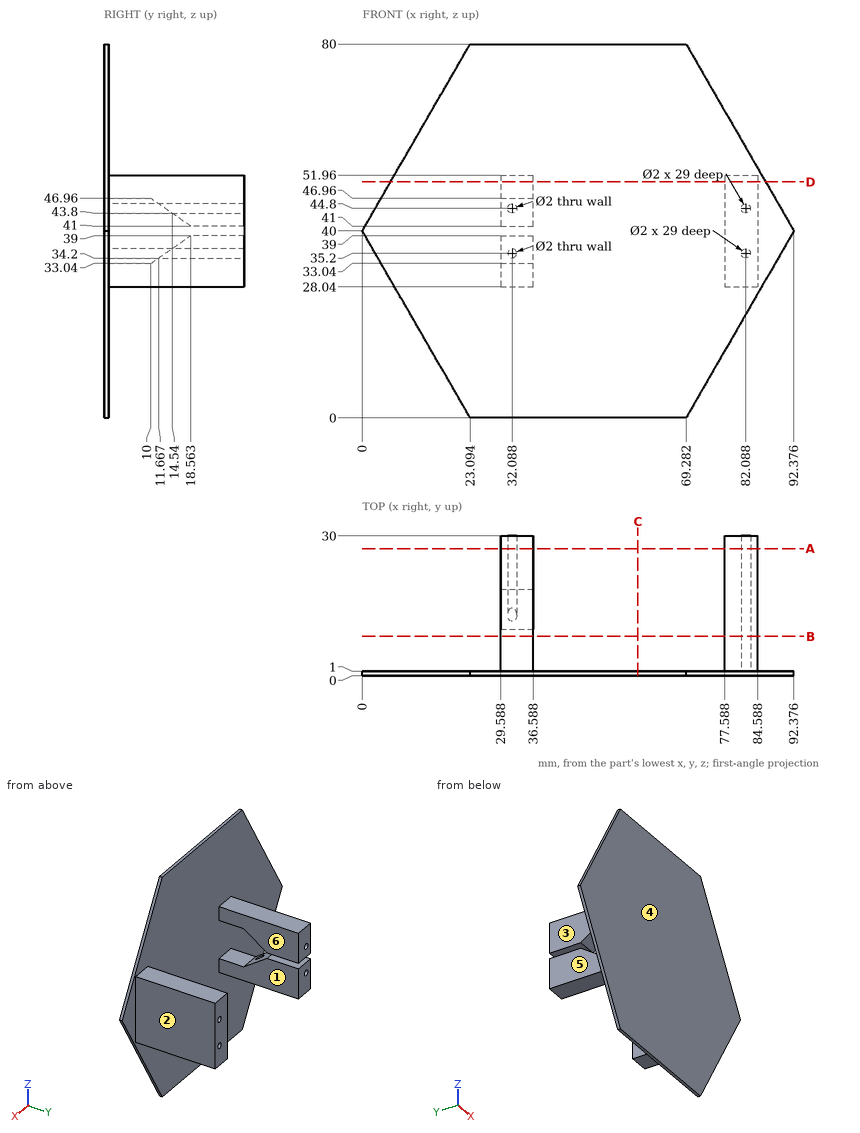
Input: dimensioned drawing with shaded views. Units: mm. Origin: part minimum x, y, z. A direction names the side the tool comes from. Give positions to 0.01 mm unless a question says otherwise; leave off trailing zeros. Write each loop counter-clockwise with the first axis right and the second up, starting at its lowest first coordinate (ties: lowest second). Pieces come first, ordered by that corner, then holes. Notation, with made-up numbers: (62, 24) -> (101, 24) arc R22 cw to (101, 43) -> close; hole circle Ø9 at (20.25, 43). An arc over 180 degrees is marked (long way). Return JSON: item names as keys, results as strings. Group by question number.
1. Pin query (flat end, axial travel): pin 1 Ø2.5 at (x, z) = (32.09, 44.8) entering from +Y; pin 2 Ø12 at (y, z) = (14.5, 37.5) entering from -X; pin 3 Ø3.5 at (x, y) = (34, 25) entering from +Z; pin 4 Ø12 at (y, z) = (10, 46.5) entering from +X. Return the tip coordinate at first contact, or that it passes through.
2. Section A-A, the plane y = 27.25. Output: boundary loops of the cut face in (x, z).
3. Section D-D, the plane z = 50.5. Output: boundary loops of the cut face in (x, y).
4. Access query for the marked faces 4, 5 and 6. Directions: +Z, -Z, +X, -X, +Y, -Y. A direction counts if a zero-diameter tool reaches every point of the face in a straight line with its end or side. Return the directions, or none.
5. Material intervals for line 1 (X direction, y = 13.5, z = 44.8); line 2 (Z direction, x = 36.5, y = 25.5); line 3 (X direction, y = 8.25, z = 35.2), sorted ascending. Write a range as from..to.
6. Section B-B, the plane y = 8.5. Output: boundary loops of the cut face in (x, z).
7. Mould query, pull axis X, two halves, no side actions, for the marked faces 1, 2 and 3. Classes: +X half, -X half, draft (parallel to the pull), parting line (faces both ways), or undercut.
8. Section C-C, the plane x = 59. Output: boundary loops of the cut face in (y, z).
Determined:
{
 "1": {"pin 1": "stops at y = 30", "pin 2": "stops at x = 29.59", "pin 3": "stops at z = 51.96", "pin 4": "stops at x = 84.59"},
 "2": {"outline": "(29.59, 28.04) -> (36.59, 28.04) -> (36.59, 39) -> (29.59, 39) -> close; (29.59, 41) -> (36.59, 41) -> (36.59, 51.96) -> (29.59, 51.96) -> close; (77.59, 28.04) -> (84.59, 28.04) -> (84.59, 51.96) -> (77.59, 51.96) -> close; hole circle Ø2 at (32.09, 35.2); hole circle Ø2 at (32.09, 44.8); hole circle Ø2 at (82.09, 35.2); hole circle Ø2 at (82.09, 44.8)"},
 "3": {"outline": "(6.06, 0) -> (86.31, 0) -> (86.31, 1) -> (84.59, 1) -> (84.59, 30) -> (77.59, 30) -> (77.59, 1) -> (36.59, 1) -> (36.59, 30) -> (29.59, 30) -> (29.59, 1) -> (6.06, 1) -> close"},
 "4": {"face 4": "+Z, -Z, +X, -X, -Y", "face 5": "+Z, -Z, -X, +Y", "face 6": "+Z, -Z, +Y"},
 "5": {"line 1": "x = 29.59..31.09, 33.09..36.59, 77.59..81.09, 83.09..84.59", "line 2": "z = 28.04..39, 41..51.96", "line 3": "x = 77.59..81.09, 83.09..84.59"},
 "6": {"outline": "(29.59, 28.04) -> (36.59, 28.04) -> (36.59, 33.04) -> (29.59, 33.04) -> close; (29.59, 46.96) -> (36.59, 46.96) -> (36.59, 51.96) -> (29.59, 51.96) -> close; (77.59, 28.04) -> (84.59, 28.04) -> (84.59, 51.96) -> (77.59, 51.96) -> close; hole circle Ø2 at (82.09, 35.2); hole circle Ø2 at (82.09, 44.8)"},
 "7": {"face 1": "undercut", "face 2": "+X half", "face 3": "-X half"},
 "8": {"outline": "(0, 0) -> (1, 0) -> (1, 80) -> (0, 80) -> close"}
}
